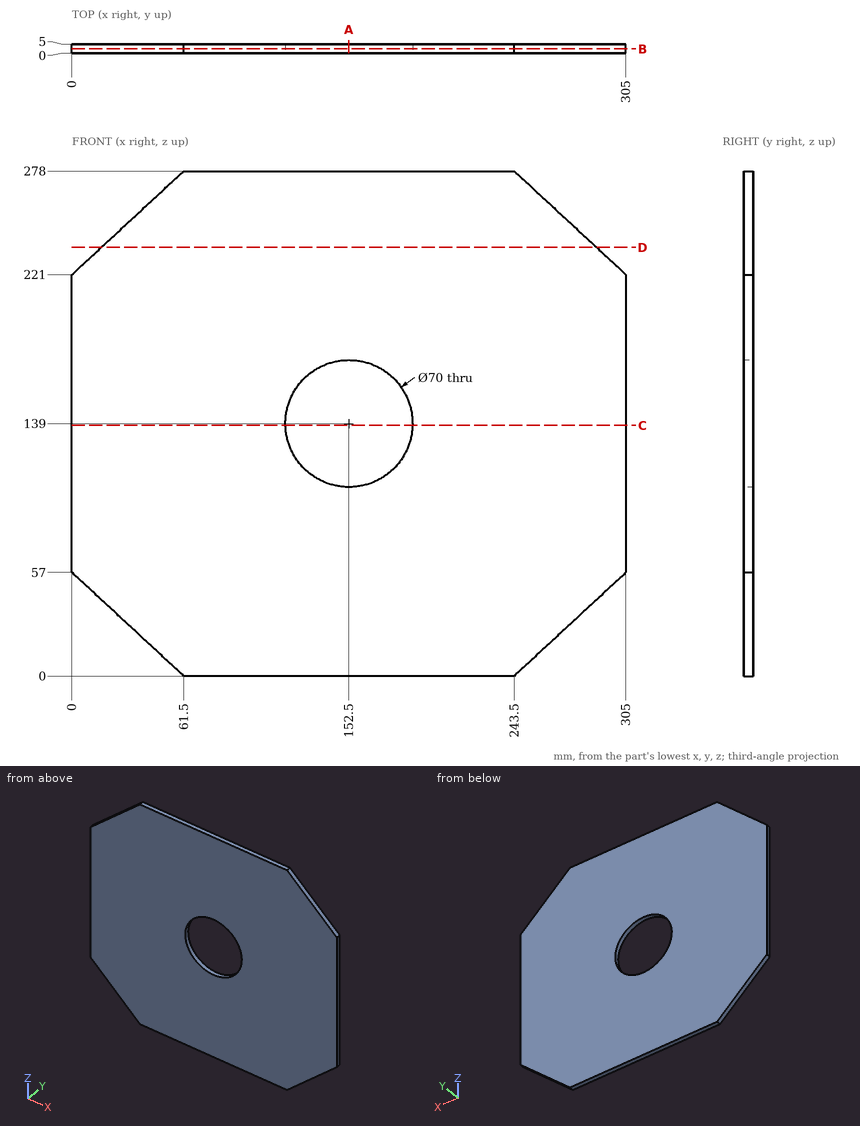
Here's the drawing with two shaded views (mm, measured from the low corner). I have some questions. Coordinates: 2 decimals unless noted, no trailing zeros. Order: outer loops, then holes, each group sorted by start corner. A loop starts at its lowest first (then second) coordinate and runs counter-clockwise, first axis right, second up.
Q1. Suppose I cut it at A-A on x = 152.5. Please give me the cut outline in (y, z).
Q2. Suppose I cut it at D-D on z = 236. Please give me the cut outline in (x, y), and give its area (3 significant figures).
Q3. Suppose I cut it at B-B on y = 2.35. Please give me the cut outline in (x, z), and give its area (3 significant figures).
Q4. Suppose I cut it at C-C on z = 138. Please give me the cut outline in (x, y).
Q5. Please list where these lines run through material, in increasing order: L1, parallel to X at y = 1.9, z = 139; L2, parallel to X at y = 3.55, z = 119; L3, parallel to Z at x = 183, y = 0.45.
Answer:
1. outline: (0, 0) - (5, 0) - (5, 104) - (0, 104) - close; (0, 174) - (5, 174) - (5, 278) - (0, 278) - close
2. outline: (16.18, 0) - (288.82, 0) - (288.82, 5) - (16.18, 5) - close
2. area: 1,360 mm2
3. outline: (0, 57) - (61.5, 0) - (243.5, 0) - (305, 57) - (305, 221) - (243.5, 278) - (61.5, 278) - (0, 221) - close; hole circle Ø70 at (152.5, 139)
3. area: 73,900 mm2
4. outline: (0, 0) - (117.51, 0) - (117.51, 5) - (0, 5) - close; (187.49, 0) - (305, 0) - (305, 5) - (187.49, 5) - close
5. L1: x = 0 to 117.5, 187.5 to 305
5. L2: x = 0 to 123.78, 181.22 to 305
5. L3: z = 0 to 121.83, 156.17 to 278
